Drawing for the job (mm, zero at the part's lowest x, y, z). Coordinates: 2 decimals unless noted, no trailing zeros. Write each loop counter-clockwise with the first axis right and the second up, starting at its lowest first coordinate (ties: lowest second). Pieces come first, ordered by that corner, then holes. Notation, with made-up numbers: (55.5, 22) - (99.5, 22) arc R32 cw to (99.5, 60) - close; hole circle Ø9 at (66.5, 15). An arc over 180 degrees is marked (long way). Write each question's results on one line, items separated by ' | '.
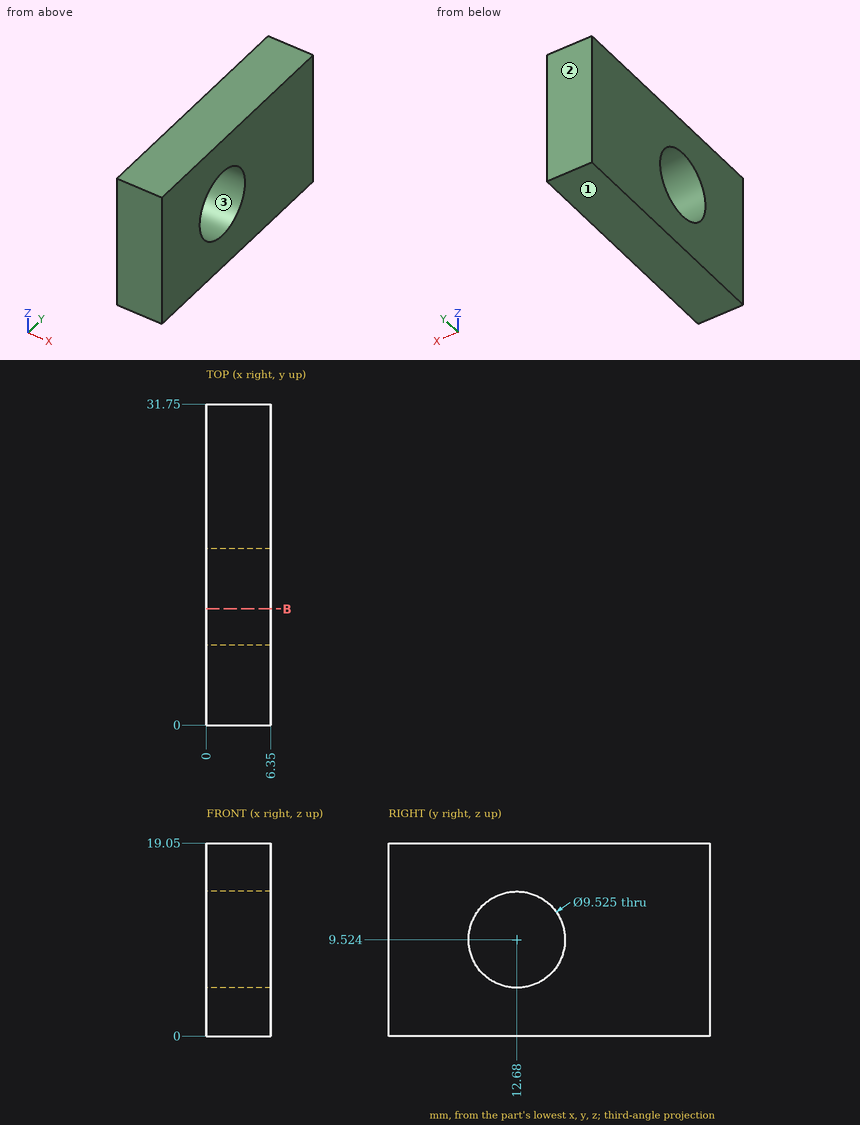
(1) Saw through at B-B on y = 11.5. Write the cut outline in (x, z).
Return value:
outline: (0, 0) - (6.35, 0) - (6.35, 4.91) - (0, 4.91) - close; (0, 14.14) - (6.35, 14.14) - (6.35, 19.05) - (0, 19.05) - close
(2) Wall check: line 1 (Y direction, x = 5, z = 9.75); line 2 (Y direction, x = 3.5, z = 11.75); line 3 (Z direction, x = 0.5, y = 14). Give the ranges that are in metal, low to high. Write a range as from..to.
Return value:
line 1: y = 0..7.92, 17.44..31.75 | line 2: y = 0..8.47, 16.89..31.75 | line 3: z = 0..4.95, 14.1..19.05
(3) Flat gauge pin, fed straight in: P1, Ø1.5, axis at y = 15, z = 7.5, coming from the -X side. Where does the tip first touch, or does it go through?
Return value:
P1: passes through
(4) Two-plate mould, pull along Z, no slides. Class the marked faces 1, 2 and 3: released by +Z, released by -Z, zero draft, split by the parting line, or undercut.
Return value:
face 1: released by -Z | face 2: zero draft | face 3: undercut
